```python
from build123d import *

# Parameters (mm, degrees)
SKETCH1_R           = 1.5
SKETCH1_R_2         = 4
BOSS_EXTRUDE1_DEPTH = 1.5


with BuildPart() as part:
    # Sketch1 → Boss-Extrude1 (new body)
    with BuildSketch(Plane(origin=(0, 0, 0), x_dir=(1, 0, 0), z_dir=(0, 1, 0))):
        with BuildLine():
            Line((-7.070663707, -8.426488874), (0, 0))
            Line((0, 0), (0, 9.381966011))
            ThreePointArc((0, 9.381966011), (-0.5, 10.5), (0, 11.618033989))
            Line((0, 11.618033989), (0, 35.5))
            Line((0, 35.5), (-15, 35.5))
            Line((-15, 35.5), (-23.677632731, 25.158400018))
            Line((-23.677632731, 25.158400018), (-129.929473623, 53.628494979))
            ThreePointArc((-129.929473623, 53.628494979), (-157.327989791, 47.078833109), (-132.17932297, 34.38547595))
            Line((-132.17932297, 34.38547595), (-33.223789423, 6.015437425))
            ThreePointArc((-33.223789423, 6.015437425), (-31.446611343, 8.081911862), (-31.03429168, 5.387719772))
            Line((-31.03429168, 5.387719772), (-23.863280614, 3.331828071))
            Line((-23.863280614, 3.331828071), (-7.070663707, -8.426488874))
        make_face()
        with Locations(Location((-8, 5.5, 0), (0, 0, 270))):
            Circle(SKETCH1_R, mode=Mode.SUBTRACT)
        with Locations(Location((-14, 15.5, 0), (0, 0, 270))):
            Circle(SKETCH1_R, mode=Mode.SUBTRACT)
        with Locations(Location((-8, 25.5, 0), (0, 0, 270))):
            Circle(SKETCH1_R, mode=Mode.SUBTRACT)
        with BuildLine():
            ThreePointArc((-143.929473623, 38.236933003), (-142.429473623, 39.736933003), (-140.929473623, 38.236933003))
            Line((-140.929473623, 38.236933003), (-140.929473623, 33.736933003))
            ThreePointArc((-140.929473623, 33.736933003), (-142.429473623, 32.236933003), (-143.929473623, 33.736933003))
            Line((-143.929473623, 33.736933003), (-143.929473623, 38.236933003))
        make_face(mode=Mode.SUBTRACT)
        with Locations(Location((-104.014603511, 35.04369958, 0), (0, 0, 270))):
            Circle(SKETCH1_R, mode=Mode.SUBTRACT)
        with BuildLine():
            ThreePointArc((-149.529473623, 46.836933003), (-148.029473623, 45.336933003), (-149.529473623, 43.836933003))
            Line((-149.529473623, 43.836933003), (-154.029473623, 43.836933003))
            ThreePointArc((-154.029473623, 43.836933003), (-155.529473623, 45.336933003), (-154.029473623, 46.836933003))
            Line((-154.029473623, 46.836933003), (-149.529473623, 46.836933003))
        make_face(mode=Mode.SUBTRACT)
        with Locations(Location((-142.429473623, 45.336933003, 0), (0, 0, 270))):
            Circle(SKETCH1_R_2, mode=Mode.SUBTRACT)
        with BuildLine():
            ThreePointArc((-135.329473623, 43.836933003), (-136.829473623, 45.336933003), (-135.329473623, 46.836933003))
            Line((-135.329473623, 46.836933003), (-130.829473623, 46.836933003))
            ThreePointArc((-130.829473623, 46.836933003), (-129.329473623, 45.336933003), (-130.829473623, 43.836933003))
            Line((-130.829473623, 43.836933003), (-135.329473623, 43.836933003))
        make_face(mode=Mode.SUBTRACT)
        with BuildLine():
            ThreePointArc((-140.929473623, 52.436933003), (-142.429473623, 50.936933003), (-143.929473623, 52.436933003))
            Line((-143.929473623, 52.436933003), (-143.929473623, 56.936933003))
            ThreePointArc((-143.929473623, 56.936933003), (-142.429473623, 58.436933003), (-140.929473623, 56.936933003))
            Line((-140.929473623, 56.936933003), (-140.929473623, 52.436933003))
        make_face(mode=Mode.SUBTRACT)
        with Locations(Location((-75.036828722, 27.279128226, 0), (0, 0, 270))):
            Circle(SKETCH1_R, mode=Mode.SUBTRACT)
    extrude(amount=BOSS_EXTRUDE1_DEPTH)


solid = part.part
```
Design review of the part built by this model. Coordinates are the model's own, in mm. A direction names the side the tool comes from. Give positions to 0.01 mm unless a question says otherwise; leave off trailing zeros. Loops run counter-clockwise (first coordinate to the right, second up) from the corner with the lowest first, then second, coordinate; pieces in that order, holes last. Notation, with made-up numbers: M -27.75,42 L 22.25,42 A28 cw 22.25,72 Z; hole C -39,68.5 d9. An arc over 180 degrees is marked long. Return JSON: item names as keys, results as strings. Group by question number.
Item 1: For probe 1 along Z at (x, y) = (-139, 0.55); probe 2 along Z at (x, y) = (-144, 0.55); probe 3 along Z at (x, y) = (-77.5, 1.4), list the stretches that pass through material, from the lowest coordinate up.
Item 2: We need section B-B (y = 0.75). Give the number of separate pieces and of enclosed holes in the cut face, and give its area (3 significant figures).
Item 3: Tool access review of faces 1 (the flat face through (-76.06, 0.74, -39.194)), 2 (the cylindrical face through (-31.493, 0.74, -8.094)): name each direction out of +Z, -Z, +X, -X, +Y, -Y from which nothing blocks a thin tool from reaching the whole face with its end or side.
Item 4: Mouldability with a two-part tool opening along X and no side actions: class faces 3 (the flat face through (-15.58, 0.74, 2.47)), 4 (the flat face through (-73, 1.5, -26)), 5 (the cylindrical face through (-103.949, 0.74, -36.542)) as released by +X, released by -X, zero draft, split by the parting line, or undercut.
Item 5: We need section C-C (x = -50.5). Give the boundary of the cut face in (y, z), and give its area (3 significant figures).
Item 6: Insertion check: pin 1 Ø0.8 at (x, y) = (-132.5, 1) entering from +Z; pin 2 Ø5 at (x, z) = (-31.86, -6.64) entering from +Y; pin 3 Ø7 at (x, z) = (-142.43, -45.34) entering from +Y. Each pin has a flat end and moves straight along its axis. Give the tip position at first contact, or say it passes through.
Item 7: We need section A-A (z = -15.5). Give the boundary of the cut face in (x, y), and give its area (3 significant figures).
Output:
{
 "1": {"probe 1": "z = -59.94 to -47.4, -43.28 to -30.73", "probe 2": "z = -60.25 to -49.02, -41.66 to -30.42", "probe 3": "z = -39.58 to -18.71"},
 "2": {"separate pieces": "1", "enclosed holes": "10", "area": "3,600 mm^2"},
 "3": {"face 1": "-Z, +Y, -Y", "face 2": "+Y, -Y"},
 "4": {"face 3": "released by -X", "face 4": "zero draft", "face 5": "undercut"},
 "5": {"outline": "M 0,-32.35 L 1.5,-32.35 L 1.5,-10.97 L 0,-10.97 Z", "area": "32.1 mm^2"},
 "6": {"pin 1": "stops at z = -33.75", "pin 2": "stops at y = 1.5", "pin 3": "passes through"},
 "7": {"outline": "M -66.31,0 L -15.5,0 L -15.5,1.5 L -66.31,1.5 Z; M -12.5,0 L 0,0 L 0,1.5 L -12.5,1.5 Z", "area": "95.0 mm^2"}
}
